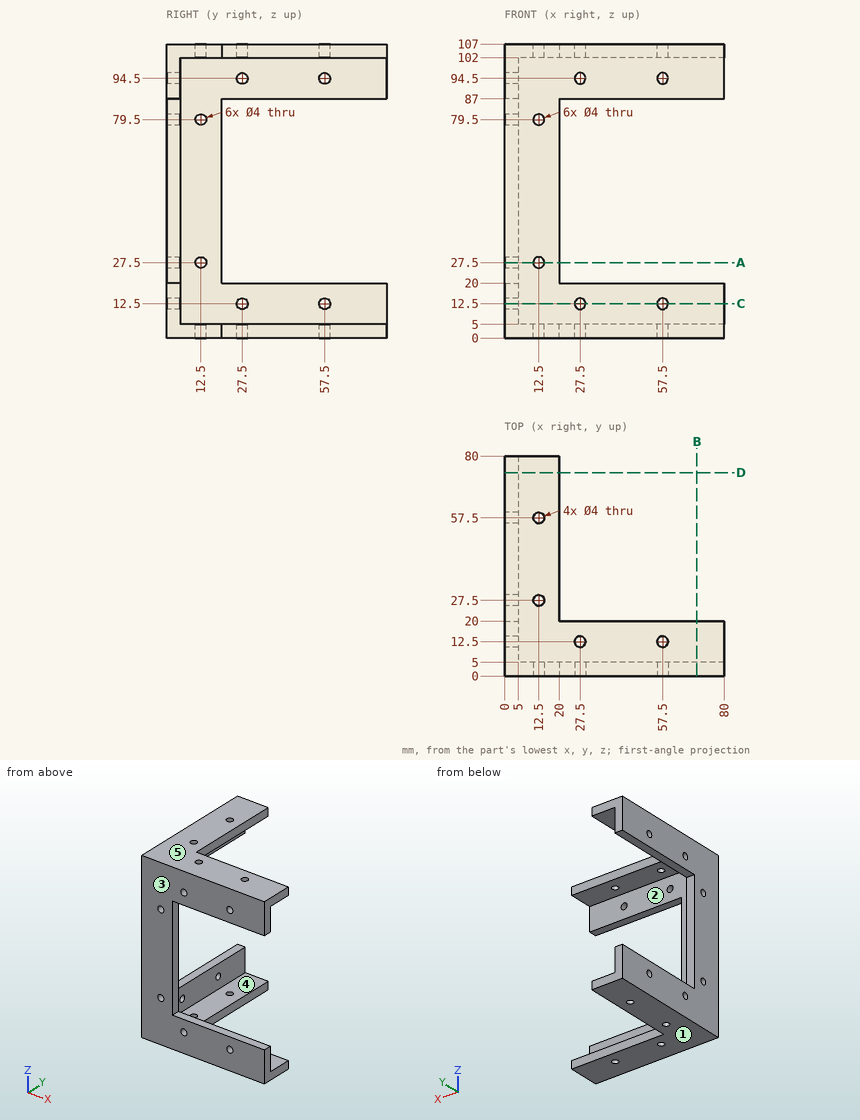
Verification items for this drawing (mm, ordinates from the low corner). A direction names the side the tool comes from. Coordinates: 2 decimals unless noted, no trailing zeros. Write each loop counter-clockwise with the first axis right and the second up, starting at its lowest first coordinate (ties: lowest second). Pieces come first, ordered by that corner, then holes. Notation, with made-up numbers: (1.25, 37) - (38.25, 37) arc R28 ccw to (38.25, 55) - close; hole circle Ø9 at (-11, -29.5). An arc over 180 degrees is marked (long way). One line per question, with ' | ' between items.
Item 1: Thickness scan on line 1 (X direction, y = 3, z = 94.5); line 2 (X direction, y = 3.3, z = 27.5); line 3 (X direction, y = 12, z = 1). Record the ranges inside material, lowest first. Write a range as [from, to].
Determined:
line 1: x = [0, 25.5], [29.5, 55.5], [59.5, 80] | line 2: x = [0, 10.5], [14.5, 20] | line 3: x = [0, 25.56], [29.44, 55.56], [59.44, 80]
Item 2: Access from +Z, -Z, +X, -X, +Y, -Y to the whole of each face (thin tool, end or side, straight path). Record for the marked faces 4 and 5.
Determined:
face 4: +X, +Y | face 5: +Z, +X, -X, +Y, -Y
Item 3: Sectioned sample at C-C on z = 12.5. Record the boundary of the cut face in (x, y).
Determined:
outline: (0, 0) - (25.5, 0) - (25.5, 5) - (5, 5) - (5, 25.5) - (0, 25.5) - close; (0, 29.5) - (5, 29.5) - (5, 55.5) - (0, 55.5) - close; (0, 59.5) - (5, 59.5) - (5, 80) - (0, 80) - close; (29.5, 0) - (55.5, 0) - (55.5, 5) - (29.5, 5) - close; (59.5, 0) - (80, 0) - (80, 5) - (59.5, 5) - close
Item 4: Sectioned sample at A-A on z = 27.5. Record the boundary of the cut face in (x, y), plus the area to 3 significant figures.
Determined:
outline: (0, 0) - (10.5, 0) - (10.5, 5) - (5, 5) - (5, 10.5) - (0, 10.5) - close; (0, 14.5) - (5, 14.5) - (5, 20) - (0, 20) - close; (14.5, 0) - (20, 0) - (20, 5) - (14.5, 5) - close | area: 135 mm2
Item 5: Gauge pin test, flat ends, axial feed: P1, Ø4, axis at x = 3, z = 45.5, coming from the +Y side; P2, Ø1.5, axis at y = 58.5, z = 90, coming from the +X side; P3, Ø2.5, axis at y = 38, z = 105, coming from the +X side. Record the tip position at first contact, or that the pin passes through.
Determined:
P1: stops at y = 20 | P2: stops at x = 5 | P3: stops at x = 20
Item 6: Mould release check, pull along Z, two halves, no side actions. Record for the marked faces 1, 2 and 3: pulls with the +Z half, pulls with the -Z half, needs draft (parallel to the pull), parting line crosses it, or undercut.
Determined:
face 1: pulls with the -Z half | face 2: undercut | face 3: needs draft
Item 7: Sectioned sample at B-B on x = 70. Record the boundary of the cut face in (y, z), plus the area to 3 significant figures.
Determined:
outline: (0, 0) - (20, 0) - (20, 5) - (5, 5) - (5, 20) - (0, 20) - close; (0, 87) - (5, 87) - (5, 102) - (20, 102) - (20, 107) - (0, 107) - close | area: 350 mm2
